from build123d import *

# Parameters (mm, degrees)
BOSS_EXTRUDE1_DEPTH = 5
SKETCH4_R           = 7
SKETCH4_R_2         = 7.5
CUT_EXTRUDE1_DEPTH  = 10


with BuildPart() as part:
    # Sketch3 → Boss-Extrude1 (new body)
    with BuildSketch(Plane(origin=(0, 0, 0), x_dir=(1, 0, 0), z_dir=(0, 1, 0))):
        with BuildLine():
            Line((-115.540454706, 15), (14.459545294, 10))
            ThreePointArc((14.459545294, 10), (24.459545294, 0), (14.459545294, -10))
            Line((14.459545294, -10), (-115.540454706, -15))
            ThreePointArc((-115.540454706, -15), (-130.540454706, 0), (-115.540454706, 15))
        make_face()
    extrude(amount=BOSS_EXTRUDE1_DEPTH)

    # Sketch4 → Cut-Extrude1 (cut)
    with BuildSketch(Plane.XZ):
        with Locations(Location((14.459545294, 0, 0), (0, 0, 270))):
            Circle(SKETCH4_R)
        with Locations(Location((-115.540454706, 0, 0), (0, 0, 270))):
            Circle(SKETCH4_R_2)
    extrude(amount=-CUT_EXTRUDE1_DEPTH, mode=Mode.SUBTRACT)


solid = part.part
The listing builds one solid part. Answer for the finished solid, in the listing's coordinates (mm). Round coordinates to 2 decimals unless told otherwise and drop trailing zeros. Loops run counter-clockwise (first coordinate to the right, second up) from the corner with the lowest first, then second, coordinate; pieces in that order, holes last. Notation, with made-up numbers: M 18,84 L 55,84 A24 ccw 55,94 Z; hole C 61.25,16.25 d3. An arc over 180 degrees is marked long. Return JSON: item names as keys, results as strings.
Q1. Find the intervals of material crossed by line 1 along X through (y, z) = (3.4, 0); line 2 along X through (y, z) = (4.4, 0.5); line 3 along Z through (x, y) = (13.5, 4.85), in increasing order. Write a range as from..to.
Results list:
{"line 1": "x = -130.54..-123.04, -108.04..7.46, 21.46..24.46", "line 2": "x = -130.53..-123.02, -108.06..7.48, 21.44..24.45", "line 3": "z = -10.04..-6.93, 6.93..10.04"}
Q2. Find section C-C, the plane y = 2.45. Determine the outline of the cut face in (x, z), plus the area to 3 significant figures.
Results list:
{"outline": "M -115.54,-15 L 14.46,-10 A10 ccw 14.46,10 L -115.54,15 A15 ccw Z; hole C -115.54,0 d15; hole C 14.46,0 d14", "area": "3,430 mm2"}
Q3. Find section A-A, the plane z = 0. Determine the outline of the cut face in (x, y).
Results list:
{"outline": "M -130.54,0 L -123.04,0 L -123.04,5 L -130.54,5 Z; M -108.04,0 L 7.46,0 L 7.46,5 L -108.04,5 Z; M 21.46,0 L 24.46,0 L 24.46,5 L 21.46,5 Z"}
Q4. Find section B-B, the plane x = 10. Determine the outline of the cut face in (y, z).
Results list:
{"outline": "M 0,-10.17 L 5,-10.17 L 5,-5.4 L 0,-5.4 Z; M 0,5.4 L 5,5.4 L 5,10.17 L 0,10.17 Z"}
Q5. Find section D-D, the plane x = -85. Determine the outline of the cut face in (y, z), plus the area to 3 significant figures.
Results list:
{"outline": "M 0,-13.83 L 5,-13.83 L 5,13.83 L 0,13.83 Z", "area": "138 mm2"}
Q6. The mould has two halves that part along Z. Classify faces 1 (the face through (-122.194, 2.465, -3.461)), 2 (the face through (-69, 5, 0)), 3 (the face through (-49.63, 2.465, 12.465)), 4 (the face through (-51.45, 2.465, -12.535)): released by +Z, released by -Z, zero draft, split by the parting line, or undercut.
Results list:
{"face 1": "undercut", "face 2": "zero draft", "face 3": "released by +Z", "face 4": "released by -Z"}
Q7. This flat-tipped pin is pushed along its axis until it touches: pin 1 Ø1 at (x, y) = (-16, 4.5) entering from -Z. Where does it stop, or does it pass through?
Results list:
{"pin 1": "stops at z = -11.19"}
